Input: dimensioned drawing with shaded views. Units: mm. Origin: part minimum x, y, z. A direction names the side the tool comes from. Round coordinates to 2 decimals unless told otherwise and drop trailing zeros. Loops run counter-clockwise (first coordinate to the right, second up) from the corner with the lowest first, then second, coordinate; pieces in that order, holes last.
Item 1: Pull-direction query (Z, two-part tool) for the marked faces 1, 2 and 3; classes: released by +Z, released by -Z, zero draft, split by the parting line, or undercut.
Item 2: Section query D-D on z = 4.05. Return loops of the section in (x, y).
Item 3: Section query A-A on x = 2.15. Return loops of the section in (y, z) (3 decimals).
Item 4: Section query B-B on z = 2.15. Return loops of the section in (x, y) (3 decimals), then the cut area to 3 significant figures.
Item 5: Ray query, L1, parallel to Y at x = 0.85, z = 3.05; L2, parallel to Z at x = 2.15, y = 5.25; L3, parallel to X at y = 4.5, z = 2.4. Return the intervals inside material, ascending.
Item 6: Access query for the marked faces 4 and 5. Directions: +Z, -Z, +X, -X, +Y, -Y. A direction counts if a zero-diameter tool reaches every point of the face in a straight line with its end or side. Return the directions, or none.
Item 7: Section query C-C on y = 4.5. Return loops of the section in (x, z).
Item 8: First-contact query: P1, Ø2.5, axis at x = 2.15, z = 2.15, coming from the +Y side. Flat tip, straight axial feed; report the tip coordinate or a pass-through.
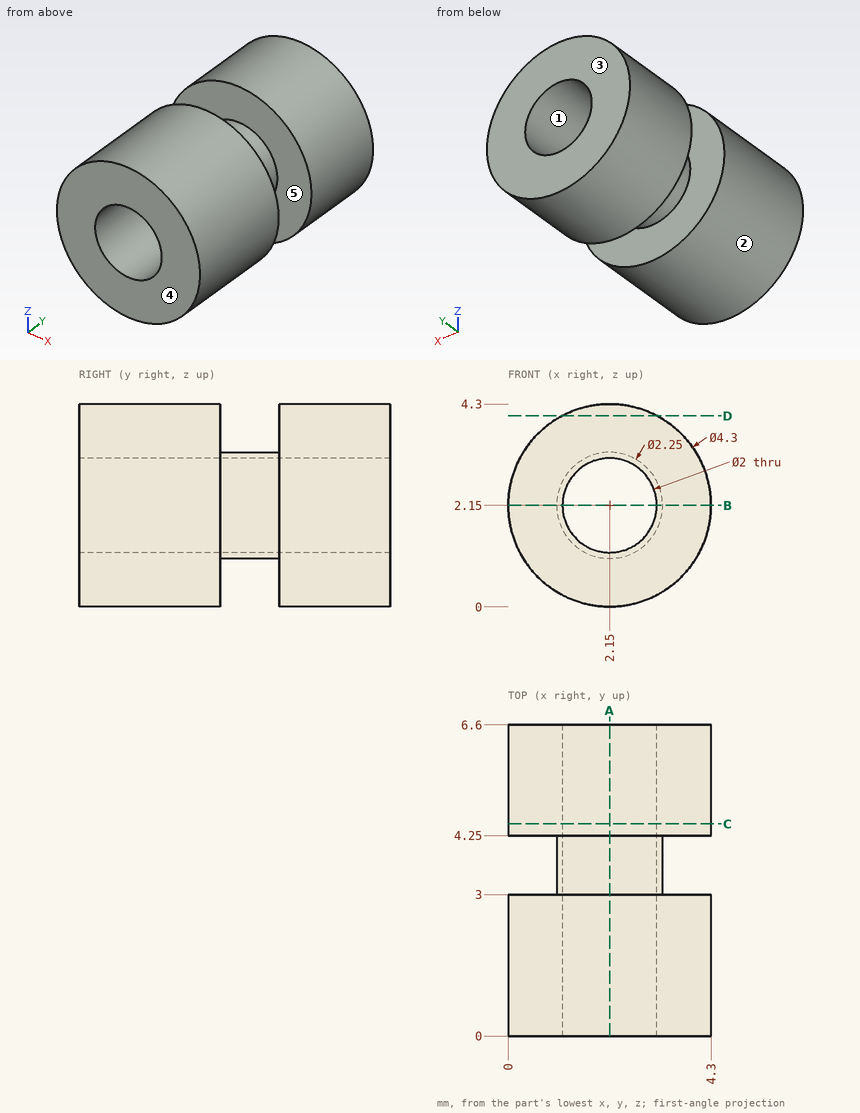
Data:
1. face 1: undercut
1. face 2: split by the parting line
1. face 3: zero draft
2. outline: (1.14, 0) - (3.16, 0) - (3.16, 3) - (1.14, 3) - close; (1.14, 4.25) - (3.16, 4.25) - (3.16, 6.6) - (1.14, 6.6) - close
3. outline: (0, 0) - (3, 0) - (3, 1.025) - (4.25, 1.025) - (4.25, 0) - (6.6, 0) - (6.6, 1.15) - (0, 1.15) - close; (0, 3.15) - (6.6, 3.15) - (6.6, 4.3) - (4.25, 4.3) - (4.25, 3.275) - (3, 3.275) - (3, 4.3) - (0, 4.3) - close
4. outline: (0, 0) - (1.15, 0) - (1.15, 6.6) - (0, 6.6) - (0, 4.25) - (1.025, 4.25) - (1.025, 3) - (0, 3) - close; (3.15, 0) - (4.3, 0) - (4.3, 3) - (3.275, 3) - (3.275, 4.25) - (4.3, 4.25) - (4.3, 6.6) - (3.15, 6.6) - close
4. area: 12.6 mm2
5. L1: y = 0 to 3, 4.25 to 6.6
5. L2: z = 0 to 1.15, 3.15 to 4.3
5. L3: x = 0.01 to 1.18, 3.12 to 4.29
6. face 4: +Z, -Z, +X, -X, -Y
6. face 5: none
7. outline: circle Ø4.3 at (2.15, 2.15); hole circle Ø2 at (2.15, 2.15)
8. P1: stops at y = 6.6
